Could you check a few things on this model? Use its own coordinates, in mm. A direction names the side the tool comes from. Coordinates: 2 decimals unless noted, no trailing zeros. Loops run counter-clockwise (first coordinate to the right, second up) from the corner with the lowest first, then second, coordinate; pieces in that order, holes last. Notation, with made-up numbers: M -34,14 L 10,14 A20 cw 10,22 Z; hole C -5.5,69.5 d2. An arc over 180 degrees is marked long. Use one line per item in the form item = value. Start each with the question number.
```python
from build123d import *

# Parameters (mm, degrees)
F1_DEPTH = 25
F3_DEPTH = 25
F4_R     = 5
F5_R     = 5
F6_R     = 5
F8_DEPTH = 25
F9_R     = 5


with BuildPart() as f1:
    # F0 (on Top) → F1 (new body)
    with BuildSketch(Plane.XY):
        Polygon((0, 38.341291), (0, 0), (-19.922435, 0), (-5.638425, 24.997016), (-40.972557, 24.997016), (-61.082937, -36.461815), (26.500596, -55.444513), (61.458834, 38.341291), align=None)
    extrude(amount=F1_DEPTH)

    # F2 (on face) → F3 (join)
    with BuildSketch(Plane(origin=(0, 0, 0), x_dir=(1, 0, 0), z_dir=(0, 0, -1))):
        Polygon((26.500596, 55.444513), (-61.082937, 36.461815), (0, 0), align=None)
        Polygon((-5.638425, -24.997016), (-19.922435, 0), (-40.972557, -24.997016), align=None)
        Polygon((61.458834, -38.341291), (47.167289, 0), (0, -38.341291), align=None)
    extrude(amount=F3_DEPTH)

    # F4
    f4_edges = [f1.edges().sort_by_distance(p)[0] for p in [
        (-30.541468, -18.230908, -25),
        (13.250298, -27.722256, -25),
        (-17.291171, -45.953164, -25),
    ]]
    fillet(f4_edges, radius=F4_R)

    # F5
    f5_edges = [f1.edges().sort_by_distance(p)[0] for p in [
        (-23.305491, 24.997016, -25),
        (-30.447496, 12.498508, -25),
        (-12.78043, 12.498508, -25),
    ]]
    fillet(f5_edges, radius=F5_R)

    # F6
    f6_edges = [f1.edges().sort_by_distance(p)[0] for p in [
        (30.729417, 38.341291, -25),
        (54.313061, 19.170646, -25),
        (23.583645, 19.170646, -25),
    ]]
    fillet(f6_edges, radius=F6_R)

    # F7 (on face) → F8 (join)
    with BuildSketch(Plane(origin=(0, 0, -25), x_dir=(1, 0, 0), z_dir=(0, 0, -1))):
        Polygon((17.59047, 48.397257), (-47.638593, 34.259627), (-10.337112, 23.305491), align=None)
    extrude(amount=F8_DEPTH)

    # F9
    f9_edges = [f1.edges().sort_by_distance(p)[0] for p in [
        (-28.987853, -28.782559, -50),
        (-15.024061, -41.328442, -50),
        (3.626679, -35.851374, -50),
    ]]
    fillet(f9_edges, radius=F9_R)


solid = f1.part
```
Item 1: I want a section at B-B (z = -39). Write out the boundary of the cut face in (x, y).
Item 2: Thinking about a two-plate mould opening in X: for faces 5 (the flat face through (23.914, 18.902, -9.86)), 6 (the flat face through (-1, -8, 25)), 7 (the flat face through (-10, 0, 12)), 8 (the flat face through (43.735, -9.208, 12.325)), which applies, pulls with the +X half, pulls with the -X half, needs draft (parallel to the pull), parting line crosses it, or undercut?
Item 3: I'm going to push flat-ended pins straight in: P1, Ø1, axis at x = -40, y = 7, coming from the -Z side; P2, Ø20, axis at y = 21.5, z = 10, coming from the -X side; P3, Ø1.5, axis at x = -35.5, y = 27, coming from the +Z side; P4, Ø1.5, axis at y = 16.5, z = 4, coming from the +X side. Where does each tip first touch, or does it pass through?
Item 4: Please list where these lines run through material, in increasing order: line 1 along Z through (x, y) = (-37.5, 14.5); line 2 along Y through (x, z) = (-37.5, -13.5); line 3 along X through (y, z) = (13, -22).
Item 5: For faces 1 (the flat face through (-37, -8, 0)), 2 (the cylindrical face through (12.079, -28.759, -23.574)), 3 (the cylindrical face through (24.15, 20.55, -23.5)), 4 (the flat face through (-8, -23, -25)), which set-ups out of +Z, -Z, +X, -X, +Y, -Y let a thin tool reach every point of the face, with its end or its side?
Item 6: I want a section at A-A (z = -11). Write out the boundary of the cut face in (x, y).
Item 7: I want a section at C-C (z = -23). Write out the boundary of the cut face in (x, y), plus the area to 3 significant figures.
Worked answers:
q1.outline = M -47.64,-34.26 L 17.59,-48.4 L -10.34,-23.31 Z
q2.face_5 = undercut
q2.face_6 = needs draft
q2.face_7 = undercut
q2.face_8 = pulls with the +X half
q3.P1 = 0
q3.P2 = -45.39
q3.P3 = through
q3.P4 = 53.6
q4.line_1 = 0 to 25
q4.line_2 = -41.57 to -22.38, 20.87 to 25
q4.line_3 = -30.32 to -12.97, 31.84 to 51.57
q5.face_1 = -Z, -X
q5.face_2 = -Z, +X
q5.face_3 = -Z
q5.face_4 = -Z, +Y
q6.outline = M -61.08,-36.46 L 26.5,-55.44 L 0,0 Z; M -40.97,25 L -19.92,0 L -5.64,25 Z; M 0,38.34 L 47.17,0 L 61.46,38.34 Z
q7.outline = M -58.39,-36.02 L 24.72,-54.04 L -0.43,-1.42 Z; M -38.82,24 L -20.08,1.74 L -7.36,24 Z; M 2.82,37.34 L 46.72,1.65 L 60.02,37.34 Z
q7.area = 3,330 mm²
